from build123d import *

# Parameters (mm, degrees)
EXTRUDE_1_DEPTH     = 230
CUT_EXTRUDE_1_DEPTH = 100


with BuildPart() as part:
    # 草图1 → 凸台-拉伸1 (new body)
    with BuildSketch(Plane.XY):
        with BuildLine():
            Line((-19, 10.5), (-14.5, 10.5))
            ThreePointArc((-14.5, 10.5), (-13.439339828, 10.060660172), (-13, 9))
            Line((-13, 9), (-13, 2))
            Line((-13, 2), (-14.5, 2))
            Line((-14.5, 2), (-14.5, 7.5))
            ThreePointArc((-14.5, 7.5), (-14.939339828, 8.560660172), (-16, 9))
            Line((-16, 9), (-17.5, 9))
            ThreePointArc((-17.5, 9), (-18.560660172, 8.560660172), (-19, 7.5))
            Line((-19, 7.5), (-19, -7.5))
            ThreePointArc((-19, -7.5), (-18.560660172, -8.560660172), (-17.5, -9))
            Line((-17.5, -9), (17.5, -9))
            ThreePointArc((17.5, -9), (18.560660172, -8.560660172), (19, -7.5))
            Line((19, -7.5), (19, 7.5))
            ThreePointArc((19, 7.5), (18.560660172, 8.560660172), (17.5, 9))
            Line((17.5, 9), (16, 9))
            ThreePointArc((16, 9), (14.939339828, 8.560660172), (14.5, 7.5))
            Line((14.5, 7.5), (14.5, 2))
            Line((14.5, 2), (13, 2))
            Line((13, 2), (13, 9))
            ThreePointArc((13, 9), (13.439339828, 10.060660172), (14.5, 10.5))
            Line((14.5, 10.5), (19, 10.5))
            ThreePointArc((19, 10.5), (20.060660172, 10.060660172), (20.5, 9))
            Line((20.5, 9), (20.5, -9))
            ThreePointArc((20.5, -9), (20.060660172, -10.060660172), (19, -10.5))
            Line((19, -10.5), (-19, -10.5))
            ThreePointArc((-19, -10.5), (-20.060660172, -10.060660172), (-20.5, -9))
            Line((-20.5, -9), (-20.5, 9))
            ThreePointArc((-20.5, 9), (-20.060660172, 10.060660172), (-19, 10.5))
        make_face()
    extrude(amount=EXTRUDE_1_DEPTH)

    # 草图3 → 切除-拉伸1 (cut)
    with BuildSketch(Plane(origin=(0, 0, 0), x_dir=(1, 0, 0), z_dir=(0, 1, 0))):
        with BuildLine():
            Line((2.5, -10), (2.5, -220))
            ThreePointArc((2.5, -220), (0, -222.5), (-2.5, -220))
            Line((-2.5, -220), (-2.5, -10))
            ThreePointArc((-2.5, -10), (0, -7.5), (2.5, -10))
        make_face()
    extrude(amount=-CUT_EXTRUDE_1_DEPTH, mode=Mode.SUBTRACT)


solid = part.part
Geometry: final body of the model. Coordinates: model frame, mm. A direction names the side the tool comes from. Coordinates: 2 decimals unless noted, no trailing zeros. Order: outer loops, then holes, each group sorted by start corner. A loop starts at its lowest first (then second) coordinate and runs counter-clockwise, first axis right, second up. Notation, with made-up numbers: M 75.25,48 L 84.25,48 A21 ccw 84.25,77 Z; hole C 17,10.25 d11. An arc over 180 degrees is marked long. One line per question, with ' | ' between items. Start each with the question number.
Item 1: Set-up query: faces 4 (the flat face through (-13, 6, 113)), 5 (the flat face through (19, 0, 113)), 6 (the flat face through (-17, 10.5, 113)). Return all of +Z, -Z, +X, -X, +Y, -Y with unobstructed straight access to the full face (end or side cutting, diameter ignored); none if empty.
Item 2: Cut plane D-D, the plane x = -9.5. Return the cut outline in (y, z).
Item 3: Draft query along X for faces 1 (the flat face through (20.5, 0, 113)), 2 (the flat face through (-19, 0, 113)), 3 (the flat face through (17, 10.5, 113)). Return one class per face: released by +X, released by -X, zero draft, split by the parting line, or undercut.
Item 4: Ray query, probe 1 along X at (y, z) = (4.75, 208); probe 2 along X at (y, z) = (-7.25, 101); probe 3 along X at (y, z) = (-9.25, 101.5). Return the intervals inside material, ascending. Write a range as [from, to].
Item 5: Pin query (flat end, axial travel): pin 1 Ø1 at (x, z) = (1.5, 205) entering from -Y (3 decimals); pin 2 Ø0.8 at (y, z) = (-9.5, 141) entering from -X; pin 3 Ø17.5 at (x, z) = (-0.5, 93.5) entering from +Y; pin 4 Ø0.8 at (y, z) = (-10, 141.5) entering from +X. Return the tip coordinate at first contact, or that it passes through.
Item 6: Cut plane C-C, the plane y = -3.25. Return the cut outline in (x, z).
Item 7: Cut plane B-B, the plane x = 0. Return the cut outline in (y, z), then the cut area to 3 significant figures.
A:
1) face 4: +Z, -Z, +Y | face 5: +Z, -Z | face 6: +Z, -Z, +X, -X, +Y
2) outline: M -10.5,0 L -9,0 L -9,230 L -10.5,230 Z
3) face 1: released by +X | face 2: undercut | face 3: zero draft
4) probe 1: x = [-20.5, -19], [-14.5, -13], [13, 14.5], [19, 20.5] | probe 2: x = [-20.5, -19], [19, 20.5] | probe 3: x = [-20.48, -2.5], [2.5, 20.48]
5) pin 1: passes through | pin 2: stops at x = -20.5 | pin 3: stops at y = -9 | pin 4: stops at x = 20.37
6) outline: M -20.5,0 L -19,0 L -19,230 L -20.5,230 Z; M 19,0 L 20.5,0 L 20.5,230 L 19,230 Z
7) outline: M -10.5,0 L -9,0 L -9,7.5 L -10.5,7.5 Z; M -10.5,222.5 L -9,222.5 L -9,230 L -10.5,230 Z | area: 22.5 mm2
